```python
from build123d import *

# Parameters (mm, degrees)
SKETCH1_W                  = 20.72
SKETCH1_H                  = 2.5
BOSS_EXTRUDE1_DEPTH        = 8.5
SKETCH2_W                  = 0.635
SKETCH2_H                  = 0.635
CUT_EXTRUDE1_DEPTH         = 6.35
CHAMFER1_SIZE              = 0.508
LPATTERN1_COUNT            = 8
LPATTERN1_PITCH            = 2.54
CHAMFER1_OF_LPATTERN1_SIZE = 0.508


with BuildPart() as part:
    # Sketch1 → Boss-Extrude1 (new body)
    with BuildSketch(Plane(origin=(0, 0, 0), x_dir=(1, 0, 0), z_dir=(0, 1, 0))):
        with Locations((10.36, 1.25)):
            Rectangle(SKETCH1_W, SKETCH1_H)
    extrude(amount=BOSS_EXTRUDE1_DEPTH)

    # Sketch2 → Cut-Extrude1 (cut)
    with BuildSketch(Plane(origin=(0, 8.5, 0), x_dir=(1, 0, 0), z_dir=(0, 1, 0))):
        with Locations((1.47, 1.25)):
            Rectangle(SKETCH2_W, SKETCH2_H)
    cut_extrude1 = extrude(amount=-CUT_EXTRUDE1_DEPTH, mode=Mode.SUBTRACT)

    # Chamfer1
    chamfer1_edges = [part.edges().sort_by_distance(p)[0] for p in [
        (1.7875, 8.5, -1.25),
        (1.47, 8.5, -1.5675),
        (1.1525, 8.5, -1.25),
        (1.47, 8.5, -0.9325),
    ]]
    chamfer(chamfer1_edges, length=CHAMFER1_SIZE)

    # LPattern1: Cut-Extrude1 ×8
    with Locations(*[(i * LPATTERN1_PITCH, 0, 0) for i in range(1, LPATTERN1_COUNT)]):
        add(cut_extrude1, mode=Mode.SUBTRACT)

    # Chamfer1 of LPattern1
    chamfer1_of_lpattern1_edges = [part.edges().sort_by_distance(p)[0] for p in [
        (4.3275, 8.5, -1.25),
        (4.01, 8.5, -1.5675),
        (3.6925, 8.5, -1.25),
        (4.01, 8.5, -0.9325),
        (6.8675, 8.5, -1.25),
        (6.55, 8.5, -1.5675),
        (6.2325, 8.5, -1.25),
        (6.55, 8.5, -0.9325),
        (9.4075, 8.5, -1.25),
        (9.09, 8.5, -1.5675),
        (8.7725, 8.5, -1.25),
        (9.09, 8.5, -0.9325),
        (11.9475, 8.5, -1.25),
        (11.63, 8.5, -1.5675),
        (11.3125, 8.5, -1.25),
        (11.63, 8.5, -0.9325),
        (14.4875, 8.5, -1.25),
        (14.17, 8.5, -1.5675),
        (13.8525, 8.5, -1.25),
        (14.17, 8.5, -0.9325),
        (17.0275, 8.5, -1.25),
        (16.71, 8.5, -1.5675),
        (16.3925, 8.5, -1.25),
        (16.71, 8.5, -0.9325),
        (19.5675, 8.5, -1.25),
        (19.25, 8.5, -1.5675),
        (18.9325, 8.5, -1.25),
        (19.25, 8.5, -0.9325),
    ]]
    chamfer(chamfer1_of_lpattern1_edges, length=CHAMFER1_OF_LPATTERN1_SIZE)


solid = part.part
```
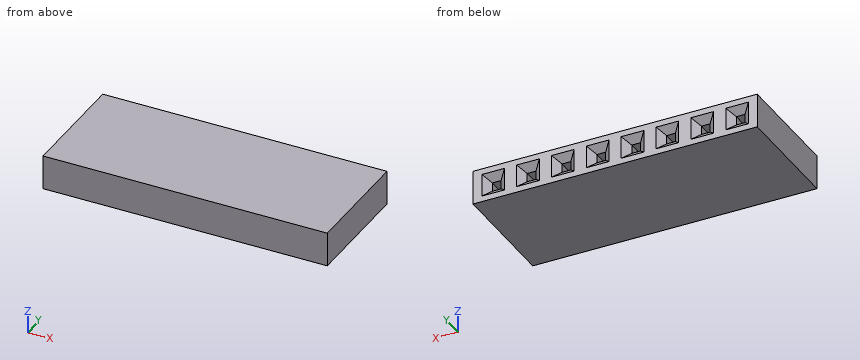
For this review, take the finished solid that the model builds, in its own axes (mm). Round coordinates to 2 decimals unless told otherwise and drop trailing zeros. Write each loop counter-clockwise with the first axis right and the second up, starting at its lowest first coordinate (ties: lowest second). Pieces come first, ordered by that corner, then holes.
1) For line 1 along Z through (x, y) = (14.25, 3.25); line 2 along Y through (x, z) = (14, -1.45); line 3 along Y through (x, z) = (9.75, -1.65), list the stretches that pass through material, from the lowest coordinate up.
Answer below:
line 1: z = -2.5 to -1.57, -0.93 to 0
line 2: y = 0 to 2.15
line 3: y = 0 to 8.33
2) Take a section at D-D on x = 6. Give the boundary of the cut face in (y, z).
Answer below:
outline: (0, -2.5) - (8.5, -2.5) - (8.5, -2.08) - (8.22, -1.8) - (8.22, -0.7) - (8.5, -0.42) - (8.5, 0) - (0, 0) - close
3) Take a section at B-B on y = 5.75. State how many separate pieces and enclosed holes the cut face has, then the cut area to 3 significant figures.
Answer below:
separate pieces: 1
enclosed holes: 8
area: 48.6 mm2
4) Take a section at A-A on x = 9. Give the boundary of the cut face in (y, z).
Answer below:
outline: (0, -2.5) - (8.5, -2.5) - (8.5, -2.08) - (7.99, -1.57) - (2.15, -1.57) - (2.15, -0.93) - (7.99, -0.93) - (8.5, -0.42) - (8.5, 0) - (0, 0) - close
5) Take a section at C-C on x = 17.25. Give the boundary of the cut face in (y, z), then the cut area to 3 significant figures.
Answer below:
outline: (0, -2.5) - (8.5, -2.5) - (8.5, -2.08) - (8.21, -1.79) - (8.21, -0.71) - (8.5, -0.42) - (8.5, 0) - (0, 0) - close
area: 20.9 mm2
